Check sheet for the drawn part. Datum: minimum x, y, z corner. Units: mm. A direction names the side the tool comes from. Coordinates: 2 decimals unless noted, no trailing zeros. Order: outer loops, then holes, each group sorted by start corner. A loop starts at its lowest first (then second) coordinate and runs counter-clockwise, first axis right, second up. Notation, with made-up numbers: (-12.75, -14.5) - (23.25, -14.5) arc R24 cw to (23.25, -2.5) - close; hole circle Ø9 at (26, 21). An arc over 180 degrees is marked (long way). Return JSON: item names as keys, results as strings. Group by question number.
Item 1: Gauge pin test, flat ends, axial feed: pin 1 (7.5 mm diameter, centred on y = 13, z = 42.5, fed in from -X); pin 2 (5 mm diameter, centred on y = 18.5, z = 39, fed in from +X); pin 3 (3 mm diameter, centred on x = 28.5, y = 3.5, fed in from +Z). Record the tip position at first contact, or that the pin passes through.
Item 2: Tool access check on the marked faces 5, 6 and 7. Record the directions out of +Z, -Z, +X, -X, +Y, -Y that give a thin tool (end or side, any length) a straight path to the whole face; none if there is none.
Item 3: Scan lines: probe 1 along Z at (x, y) = (33.5, 10.25); probe 2 along X at (y, z) = (15.5, 17.5) (1 decimal); probe 3 along X at (y, z) = (11.5, 24) (1 decimal). Record each from-to range of solid material in increasing order.
Item 4: Section check A-A on x = 9. Enter the section's corners in (y, z) (1 decimal).
Item 5: Section check B-B on z = 17.5. Enter the section's corners in (x, y), then the cut area to 3 significant figures.
Item 6: Section check C-C on y = 8.5. Enter the section's corners in (x, z).
Item 7: Section check D-D on x = 66.5. Enter the section's corners in (y, z).
Item 8: Draft check along X on the marked faces 1, 2, 3 and 4. Enter one of: pulls with the +X half, pulls with the -X half, needs draft (parallel to the pull), parting line crosses it, or undercut.
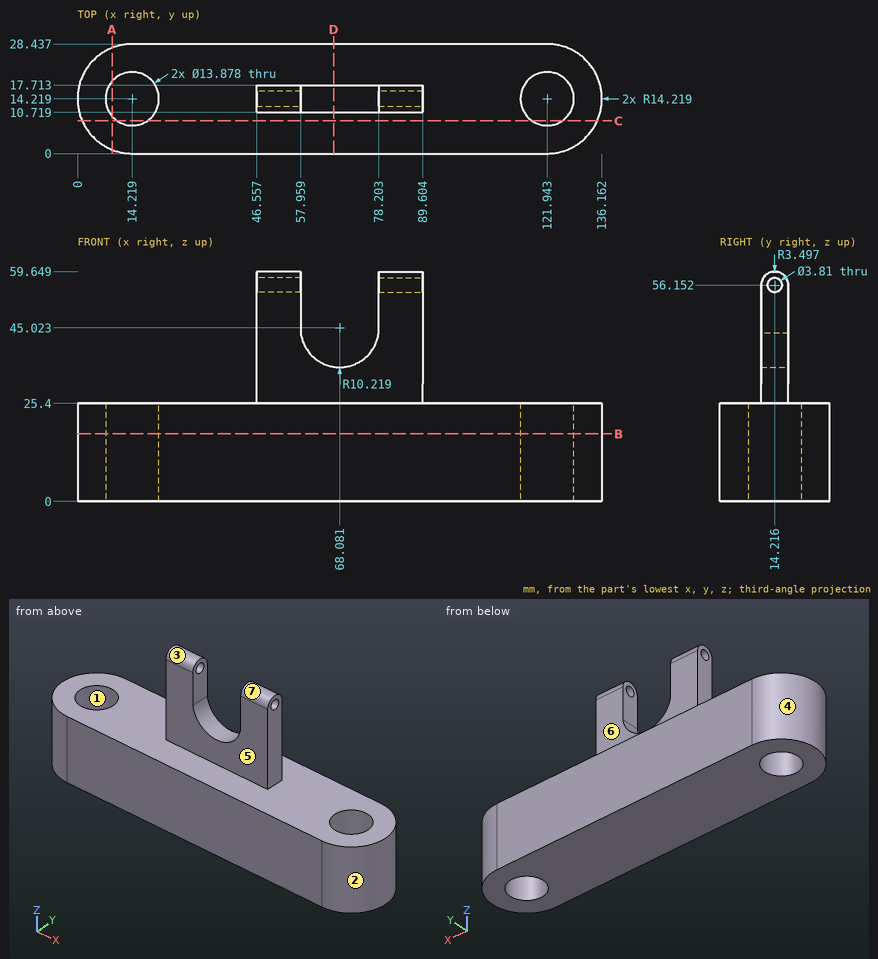
Computed:
{
 "1": {"pin 1": "stops at x = 46.56", "pin 2": "stops at x = 89.6", "pin 3": "stops at z = 25.4"},
 "2": {"face 5": "+Z, +X, -X, -Y", "face 6": "+Z, +X, -X, +Y", "face 7": "+Z, +X, -X"},
 "3": {"probe 1": "z = 0 to 25.4", "probe 2": "x = 0.1 to 7.4, 21 to 115.1, 128.8 to 136.1", "probe 3": "x = 0.3 to 7.8, 20.6 to 115.6, 128.3 to 135.9"},
 "4": {"outline": "(1, 0) - (9.6, 0) - (9.6, 25.4) - (1, 25.4) - close; (18.8, 0) - (27.4, 0) - (27.4, 25.4) - (18.8, 25.4) - close"},
 "5": {"outline": "(14.22, 0) - (121.94, 0) arc R14.22 ccw to (121.94, 28.44) - (14.22, 28.44) arc R14.22 ccw to start; hole circle Ø13.88 at (14.22, 14.22); hole circle Ø13.88 at (121.94, 14.22)", "area": "3,400 mm²"},
 "6": {"outline": "(1.2, 0) - (10.29, 0) - (10.29, 25.4) - (1.2, 25.4) - close; (18.15, 0) - (118.01, 0) - (118.01, 25.4) - (18.15, 25.4) - close; (125.87, 0) - (134.96, 0) - (134.96, 25.4) - (125.87, 25.4) - close"},
 "7": {"outline": "(0, 0) - (28.44, 0) - (28.44, 25.4) - (17.71, 25.4) - (17.71, 34.93) - (10.72, 34.93) - (10.72, 25.4) - (0, 25.4) - close"},
 "8": {"face 1": "undercut", "face 2": "pulls with the +X half", "face 3": "needs draft", "face 4": "pulls with the -X half"}
}
